Design review of the part built by this model. Coordinates are the model's own, in mm. Round coordinates to 2 decimals unless told otherwise and drop trailing zeros. Loops run counter-clockwise (first coordinate to the right, second up) from the corner with the lowest first, then second, coordinate; pieces in that order, holes last. Notation, with made-up numbers: (68.25, 1.5) - (127.25, 1.5) arc R36 ccw to (127.25, 36.5) - close; hole circle Ø1 at (86, -38.5). An arc over 180 degrees is marked (long way). Return JSON: item names as keys, results as strings. Group by question number.
from build123d import *

# Parameters (mm, degrees)
SKETCH_1_R      = 7.5
EXTRUDE_1_DEPTH = 30


with BuildPart() as part:
    # Эскиз1 → Бобышка-Вытянуть1 (new body)
    with BuildSketch(Plane.XY):
        Circle(SKETCH_1_R)
        with BuildLine():
            Line((0, 5.579989869), (0, 4))
            ThreePointArc((0, 4), (-0.62573786, 3.950753362), (-1.236067977, 3.804226065))
            Line((-1.236067977, 3.804226065), (-1.724311698, 5.306885726))
            ThreePointArc((-1.724311698, 5.306885726), (-2.533262389, 4.971807378), (-3.279835753, 4.514306633))
            Line((-3.279835753, 4.514306633), (-2.351141009, 3.236067977))
            ThreePointArc((-2.351141009, 3.236067977), (-2.828427125, 2.828427125), (-3.236067977, 2.351141009))
            Line((-3.236067977, 2.351141009), (-4.514306633, 3.279835753))
            ThreePointArc((-4.514306633, 3.279835753), (-4.971807378, 2.533262389), (-5.306885726, 1.724311698))
            Line((-5.306885726, 1.724311698), (-3.804226065, 1.236067977))
            ThreePointArc((-3.804226065, 1.236067977), (-3.950753362, 0.62573786), (-4, 0))
            Line((-4, 0), (-5.579989869, 0))
            ThreePointArc((-5.579989869, 0), (-5.511290934, -0.87290273), (-5.306885726, -1.724311698))
            Line((-5.306885726, -1.724311698), (-3.804226065, -1.236067977))
            ThreePointArc((-3.804226065, -1.236067977), (-3.564026097, -1.815961999), (-3.236067977, -2.351141009))
            Line((-3.236067977, -2.351141009), (-4.514306633, -3.279835753))
            ThreePointArc((-4.514306633, -3.279835753), (-3.945648675, -3.945648675), (-3.279835753, -4.514306633))
            Line((-3.279835753, -4.514306633), (-2.351141009, -3.236067977))
            ThreePointArc((-2.351141009, -3.236067977), (-1.815961999, -3.564026097), (-1.236067977, -3.804226065))
            Line((-1.236067977, -3.804226065), (-1.724311698, -5.306885726))
            ThreePointArc((-1.724311698, -5.306885726), (-0.87290273, -5.511290934), (0, -5.579989869))
            Line((0, -5.579989869), (0, -4))
            ThreePointArc((0, -4), (0.62573786, -3.950753362), (1.236067977, -3.804226065))
            Line((1.236067977, -3.804226065), (1.724311698, -5.306885726))
            ThreePointArc((1.724311698, -5.306885726), (2.533262389, -4.971807378), (3.279835753, -4.514306633))
            Line((3.279835753, -4.514306633), (2.351141009, -3.236067977))
            ThreePointArc((2.351141009, -3.236067977), (2.828427125, -2.828427125), (3.236067977, -2.351141009))
            Line((3.236067977, -2.351141009), (4.514306633, -3.279835753))
            ThreePointArc((4.514306633, -3.279835753), (4.971807378, -2.533262389), (5.306885726, -1.724311698))
            Line((5.306885726, -1.724311698), (3.804226065, -1.236067977))
            ThreePointArc((3.804226065, -1.236067977), (3.950753362, -0.62573786), (4, 0))
            Line((4, 0), (5.579989869, 0))
            ThreePointArc((5.579989869, 0), (5.511290934, 0.87290273), (5.306885726, 1.724311698))
            Line((5.306885726, 1.724311698), (3.804226065, 1.236067977))
            ThreePointArc((3.804226065, 1.236067977), (3.564026097, 1.815961999), (3.236067977, 2.351141009))
            Line((3.236067977, 2.351141009), (4.514306633, 3.279835753))
            ThreePointArc((4.514306633, 3.279835753), (3.945648675, 3.945648675), (3.279835753, 4.514306633))
            Line((3.279835753, 4.514306633), (2.351141009, 3.236067977))
            ThreePointArc((2.351141009, 3.236067977), (1.815961999, 3.564026097), (1.236067977, 3.804226065))
            Line((1.236067977, 3.804226065), (1.724311698, 5.306885726))
            ThreePointArc((1.724311698, 5.306885726), (0.87290273, 5.511290934), (0, 5.579989869))
        make_face(mode=Mode.SUBTRACT)
    extrude(amount=EXTRUDE_1_DEPTH)


solid = part.part
Q1. Add section A-A, the plane y = 6.5. State the section outline as (x, z) points.
Q2. Draft analysis for pull direction Y (two halves, no side actions). For faces 1 (the flat face through (3, -3, 0)), 2 (the flat face through (3.87, 2.81, 14.79)), state which applies: pulls with the +Y half, pulls with the -Y half, needs draft (parallel to the pull), parting line crosses it, or undercut.
Q3. Insertion check: pin 1 Ø0.8 at (x, z) = (-4.5, 17) entering from -Y; pin 2 Ø1 at (x, z) = (2, 8) entering from -Y; pin 3 Ø0.8 at (y, z) = (-5, 13.5) entering from -X. Each pin has a flat end and moves straight along its axis. Give the tip position at first contact, or say it passes through.
Q4. For line 1 (Y direction, x = -0.25, z = 13); line 2 (Y direction, x = 2.75, z = 1.5); line 3 (Y direction, x = -2.75, z = 24), list the stretches that pass through material, from the lowest coordinate up.
Evaluation:
{
 "1": {"outline": "(-3.74, 0) - (3.74, 0) - (3.74, 30) - (-3.74, 30) - close"},
 "2": {"face 1": "needs draft", "face 2": "undercut"},
 "3": {"pin 1": "y = -6.28", "pin 2": "y = -7.35", "pin 3": "x = -5.92"},
 "4": {"line 1": "-7.5 to -5.57, 3.99 to 7.5", "line 2": "-6.98 to -4.86, -3.79 to -2.9, 3.79 to 6.98", "line 3": "-6.98 to -3.79, 2.9 to 3.79, 4.86 to 6.98"}
}
